Autodesk Inventor part; units mm, degrees
ref_plane "YZ Plane" through (0, 0, 0) normal (1, 0, 0) x (0, 1, 0)
ref_plane "XZ Plane" through (0, 0, 0) normal (0, 1, 0) x (-1, 0, 0)
ref_plane "XY Plane" through (0, 0, 0) normal (0, 0, 1) x (1, 0, 0)
sketch "Эскиз1" plane through (0, 0, 0) normal (0, 0, 1) x (1, 0, 0)
  line L0 (112.2275, 7.2678) -> (167.2275, 7.2678)
  line L1 (167.2275, 7.2678) -> (167.2275, -32.7322)
  line L2 (167.2275, -32.7322) -> (112.2275, -32.7322)
  line L3 (112.2275, -32.7322) -> (112.2275, 7.2678)
  line L4 (112.2275, 7.2678) -> (167.2275, -32.7322) construction
  line L5 (167.2275, 7.2678) -> (112.2275, -32.7322) construction
  line L6 (147.2275, -32.7322) -> (167.2275, -32.7322)
  point P0 (139.7275, -12.7322)
  point P1 (139.7275, -32.7322)
  dimension "d55" = 40
  dimension "d67" = 55
extrude "Выдавливание1" add sketch "Эскиз1" along normal blind 4
sketch "Эскиз6" plane through (0, 0, 4) normal (0, 0, 1) x (1, 0, 0)
  line L0 (112.2275, -32.7322) -> (167.2275, -32.7322) construction
  line L1 (167.2275, 7.2678) -> (112.2275, 7.2678) construction
  line L2 (112.2275, 7.2678) -> (112.2275, -32.7322) construction
  circle A0 centre (120.2275, 0.5528) radius 2.65
  line L3 (167.2275, -32.7322) -> (167.2275, 7.2678)
  line L4 (112.2275, -32.7322) -> (167.2275, -32.7322)
  line L5 (139.7275, -32.7322) -> (139.7275, 7.2678) construction
  circle A1 centre (159.2275, 0.5528) radius 2.65
  line L6 (167.2275, 7.2678) -> (112.2275, 7.2678)
  line L7 (112.2275, 7.2678) -> (112.2275, -32.7322)
  circle A2 centre (120.2275, -7.0322) radius 2.65
  circle A3 centre (159.2275, -7.0322) radius 2.65
  point P0 (0, 0)
  dimension "d76" = 8
  dimension "d77" = 5.3
  dimension "d78" = 6.715
  dimension "d79" = 5.3
  dimension "d80" = 14.3
extrude "Выдавливание5" cut sketch "Эскиз6" against normal blind 4 contours A0 | A1 | A2 | A3
fillet "Сопряжение5" radius 4 4 edges at (112.2275, -32.7322, 2) (112.2275, 7.2678, 2) (167.2275, 7.2678, 2) (167.2275, -32.7322, 2)
properties part number "креп_центр_рейки"
For this review, take the finished solid that the model builds, in its own axes (mm). Round coordinates to 2 decimals unless told otherwise and drop trailing zeros. Write each loop counter-clockwise with the first axis right and the second up, starting at its lowest first coordinate (ties: lowest second). Pieces come first, ordered by that corner, then holes. Notation, with made-up numbers: (30.5, 50) - (40.5, 50) arc R33 cw to (40.5, 83) - close; hole circle Ø6 at (54, 3). An arc over 180 degrees is marked (long way). Write each question's results on one line, items separated by ' | '.
Item 1: For pin 1 (5 mm diameter, centred on x = 159.23, y = 0.55, fed in from -Z), flat-tipped, find the tip position at first contact; note if it passes through.
Calculated:
pin 1: passes through
Item 2: Draft analysis for pull direction Y (two halves, no side actions). For faces 1 (the face through (113.37, -31.53, 2.03)), 2 (the face through (139, -12, 0)), 3 (the face through (161.675, -0.462, 2.028)), state which applies: pulls with the +Y half, pulls with the -Y half, needs draft (parallel to the pull), parting line crosses it, or undercut.
Calculated:
face 1: pulls with the -Y half | face 2: needs draft | face 3: undercut
Item 3: Take a section at A-A on z = 1.6. State the section outline as (x, y) points, then the cut area to 3 significant figures.
Calculated:
outline: (112.23, -28.73) arc R4 ccw to (116.23, -32.73) - (163.23, -32.73) arc R4 ccw to (167.23, -28.73) - (167.23, 3.27) arc R4 ccw to (163.23, 7.27) - (116.23, 7.27) arc R4 ccw to (112.23, 3.27) - close; hole circle Ø5.3 at (120.23, -7.03); hole circle Ø5.3 at (120.23, 0.55); hole circle Ø5.3 at (159.23, -7.03); hole circle Ø5.3 at (159.23, 0.55) | area: 2,100 mm^2
Item 4: To check wall thickness, follow line 1 along Y through (x, z) = (120, 1.25); line 2 along X through (y, z) = (1.5, 3.1); line 3 along Y through (x, z) = (118, 1.5). State the ranges of each line that lie inside material, in increasing order. Write a range as from..to.
Calculated:
line 1: y = -32.73..-9.67, -4.39..-2.09, 3.19..7.27 | line 2: x = 112.23..117.75, 122.7..156.75, 161.7..167.23 | line 3: y = -32.73..-8.47, -5.6..-0.88, 1.99..7.27
